from build123d import *

# Parameters (mm, degrees)
SKETCH1_R                = 19
BOSS_EXTRUDE1_DEPTH      = 46
SKETCH2_R                = 9.65
BOSS_EXTRUDE2_DEPTH      = 505
SKETCH3_R                = 11.15
BOSS_EXTRUDE3_DEPTH      = 250
CHAMFER1_SIZE            = 9
FILLET1_R                = 10
BOSS_EXTRUDE4_DEPTH      = 90
BOSS_EXTRUDE4_DEPTH_BACK = 50
SKETCH4_R                = 14.05
FILLET2_R                = 7


with BuildPart() as part:
    # Sketch1 → Boss-Extrude1 (new body)
    with BuildSketch(Plane(origin=(0, 0, 0), x_dir=(1, 0, 0), z_dir=(0, 1, 0))):
        with Locations(Location((0, 0, 0), (0, 0, 270))):
            Circle(SKETCH1_R)
    extrude(amount=BOSS_EXTRUDE1_DEPTH)

    # Sketch2 → Boss-Extrude2 (add)
    with BuildSketch(Plane(origin=(0, 46, 0), x_dir=(1, 0, 0), z_dir=(0, 1, 0))):
        with Locations(Location((0, 0, 0), (0, 0, 270))):
            Circle(SKETCH2_R)
    extrude(amount=BOSS_EXTRUDE2_DEPTH)

    # Sketch3 → Boss-Extrude3 (add)
    with BuildSketch(Plane(origin=(0, 551, 0), x_dir=(1, 0, 0), z_dir=(0, 1, 0))):
        with Locations(Location((0, 0, 0), (0, 0, 270))):
            Circle(SKETCH3_R)
    extrude(amount=BOSS_EXTRUDE3_DEPTH)

    # Chamfer1
    chamfer1_edges = [part.edges().sort_by_distance(p)[0] for p in [
        (0, 46, -9.65),
    ]]
    chamfer(chamfer1_edges, length=CHAMFER1_SIZE)

    # Fillet1
    # the kernel refuses this fillet: 10 mm, written as the material it takes off along each edge
    with BuildSketch(Plane(origin=(0, 551, 0), x_dir=(0, 0, 1), z_dir=(-1, 0, 0))) as fillet1_piece_1:
        with BuildLine():
            CenterArc((1.15, 5.267826876), FILLET1_R, 328.211669383, 31.788330617)
            Line((11.15, 5.267826876), (11.35, 5.267826876))
            Line((11.35, 5.267826876), (11.35, 0))
            Line((11.35, 0), (11.15, -0.2))
            ThreePointArc((11.15, -0.2), (10.4, -0.2), (9.82, -0.105356538))
            Line((9.82, -0.105356538), (9.65, 0))
        make_face()
    revolve(axis=Axis((0, 551, 0), (0, 1, 0)), mode=Mode.SUBTRACT)

    # Sketch4 → Boss-Extrude4 (add, two sides: drawn at the far end of the back side and taken through both)
    with BuildSketch(Plane.XY.offset(-BOSS_EXTRUDE4_DEPTH_BACK)):
        with Locations((0, 809)):
            Circle(SKETCH4_R)
    extrude(amount=BOSS_EXTRUDE4_DEPTH + BOSS_EXTRUDE4_DEPTH_BACK)

    # Fillet2
    fillet2_edges = [part.edges().sort_by_distance(p)[0] for p in [
        (-14.05, 809, -50),
        (-14.05, 809, 90),
    ]]
    fillet(fillet2_edges, radius=FILLET2_R)


solid = part.part
Source: CAD feature listing. Evaluate the final solid. Frame: model axes, mm. A direction names the side the tool comes from. Round coordinates to 2 decimals unless told otherwise and drop trailing zeros. Order: outer loops, then holes, each group sorted by start corner. A loop starts at its lowest first (then second) coordinate and runs counter-clockwise, first axis right, second up. Notation, with made-up numbers: (76.25, 6) - (114.25, 6) arc R7 ccw to (114.25, 14) - close; hole circle Ø5 at (59.25, -26). An arc over 180 degrees is marked (long way). Use a Markdown table: item, result. Add a question column.
1. Mould query, pull axis Y, two halves, no side actions, for faces 1 (the flat face through (0, 809, 90)), 2 (the flat face through (0, 0, 0)), 3 (the cylindrical face through (-10.885, 676.65, -2.417)). Classes: +Y half, -Y half, draft (parallel to the pull), parting line (faces both ways), or undercut.
2. Line query: probe 1 along Y at (x, z) = (1, -1); probe 2 along Z at (x, y) = (1, 63.5); probe 3 along Y at (x, z) = (-0.5, 38). Output: solid intervals per line, ascending.
3. Section query A-A (z = 68). Return the cut outline in (x, y).
4. First-contact query: pin 1 (8 mm diameter, centred on x = 8, z = 3, fed in from +Y); pin 2 (8 mm diameter, centred on x = 15, z = -27, fed in from +Y); pin 3 (2 mm diameter, centred on x = -2, z = 32, fed in from -Y); pin 4 (10 mm diameter, centred on x = -0.5, z = 53, fed in from +Y). Flat tips, straight axial feed; report the tip coordinate or a pass-through.
5. Set-up query: faces 4 (the cylindrical face through (-11.56, 22.68, -15.08)), 5 (the flat face through (0, 809, -50)), 6 (the conical face through (-9.97, 54.44, -2.21)). Return all of +Z, -Z, +X, -X, +Y, -Y with unobstructed straight access to the full face (end or side cutting, diameter ignored); none if empty.
6. Section query B-B (y = 517). Return the cut outline in (x, z), then the cut area to 3 significant figures.
Derived:
| question | item | result |
|---|---|---|
| 1 | face 1 | draft |
| 1 | face 2 | -Y half |
| 1 | face 3 | undercut |
| 2 | probe 1 | 0 to 823.01 |
| 2 | probe 2 | -9.6 to 9.6 |
| 2 | probe 3 | 794.96 to 823.04 |
| 3 | outline | circle Ø28.1 at (0, 809) |
| 4 | pin 1 | y = 822.47 |
| 4 | pin 2 | y = 817.74 |
| 4 | pin 3 | y = 794.99 |
| 4 | pin 4 | y = 823.05 |
| 5 | face 4 | -Y |
| 5 | face 5 | -Z, +X, -X, +Y, -Y |
| 5 | face 6 | none |
| 6 | outline | circle Ø19.3 at (0, 0) |
| 6 | area | 293 mm2 |
